Autodesk Inventor part; units mm, degrees
ref_plane "YZ Plane" through (0, 0, 0) normal (1, 0, 0) x (0, 1, 0)
ref_plane "XZ Plane" through (0, 0, 0) normal (0, 1, 0) x (-1, 0, 0)
ref_plane "XY Plane" through (0, 0, 0) normal (0, 0, 1) x (1, 0, 0)
ref_plane "Work Plane1" through (-237.6364, -237.6364, 0) normal (0, 0, 1) x (0.7071, 0.7071, 0)
sketch "Sketch1" plane through (-237.6364, -237.6364, 0) normal (0, 0, 1) x (0.7071, 0.7071, 0)
  circle A0 centre (0, 0) radius 4.15 construction
  circle A1 centre (336.0686, 0) radius 6.45 construction
  circle A2 centre (246.0297, 47.9271) radius 4.83 construction
  circle A3 centre (102, -0.0729) radius 4.83 construction
  circle A4 centre (0, 0) radius 6.8857
  circle A5 centre (336.0686, 0) radius 6.8834
  circle A6 centre (102, -0.0729) radius 6.8834
  circle A7 centre (246.0297, 47.9271) radius 6.8834
  line L0 (78.0149, 71.9271) -> (270.0149, 71.9271) construction
  line L1 (168.0343, 78.2771) -> (168.0343, 71.9271)
  line L2 (168.0343, 78.2771) -> (393.4593, 78.2771)
  line L3 (168.0343, 78.2771) -> (-57.3907, 78.2771)
  line L4 (-57.3907, -31.75) -> (-57.3907, 78.2771)
  line L5 (-57.3907, -31.75) -> (358.1679, -31.75)
  line L6 (393.4593, 3.5414) -> (393.4593, 78.2771)
  arc A8 (358.1679, -31.75) -> (393.4593, 3.5414) centre (358.1679, 3.5414) ccw
  point P0 (336.0686, 0)
  dimension "d0" = 13.7714
  dimension "d1" = 13.7668
  dimension "d2" = 13.7668
  dimension "d3" = 13.7668
  dimension "d6" = 225.425
  dimension "d7" = 225.425
extrude "Extrusion1" add sketch "Sketch1" along normal blind 6.35
sketch "Sketch3" plane through (-237.6364, -237.6364, 6.35) normal (0, 0, 1) x (0.7071, -0.7071, 0)
  circle A0 centre (-63.9271, 166.0149) radius 3.81 construction
  circle A1 centre (-31.9271, 166.0149) radius 3.81 construction
  circle A2 centre (-15.9271, 166.0149) radius 3.81 construction
  circle A3 centre (-63.9271, 86.0149) radius 3.81 construction
  circle A4 centre (16.0729, 166.0149) radius 3.81 construction
  circle A5 centre (-31.9271, 166.0149) radius 3.81 construction
  circle A6 centre (-63.9271, 86.0149) radius 5.08 construction
  circle A7 centre (-31.9271, 86.0149) radius 3.81 construction
  circle A8 centre (-15.9271, 86.0149) radius 3.81 construction
  circle A9 centre (16.0729, 86.0149) radius 3.81 construction
  circle A10 centre (-63.9271, 86.0149) radius 1.778
  circle A11 centre (-31.9271, 166.0149) radius 1.778
  circle A12 centre (-63.9271, 166.0149) radius 1.778
  circle A13 centre (16.0729, 166.0149) radius 1.9304 construction
  circle A14 centre (16.0729, 246.0149) radius 1.9304 construction
  circle A15 centre (-15.9271, 166.0149) radius 1.9304 construction
  circle A16 centre (16.0729, 246.0149) radius 1.778
  point P0 (0, 336.0686)
  dimension "d11" = 3.556
  dimension "d17" = 3.556
  dimension "d18" = 3.556
  dimension "d21" = 3.556
extrude "Extrusion2" cut sketch "Sketch3" against normal through all contours A10 | A11 | A12
properties part number "new sidewall outside"
Part model, mm, in its own coordinate system. Round coordinates to 2 decimals unless told otherwise and drop trailing zeros. Loops run counter-clockwise (first coordinate to the right, second up) from the corner with the lowest first, then second, coordinate; pieces in that order, holes last. Notation, with made-up numbers: (39, 84) -> (75, 84) arc R24 cw to (75, 102) -> close; hole circle Ø7 at (61, 26). An arc over 180 degrees is marked (long way). Use one line per item in the form item = value. Start each with the question number.
Item 1: Band-saw the part on A-A (x = -240). List the corners of the cut face in (y, z), plus the area to 3 significant figures.
Item 2: Two-plate mould, pull along X, no slides. Class faces 1 (the cylindrical face through (-97.855, -36.655, 3.131)), 2 (the flat face through (-176.4, -65.7, 3.1)), 3 (the cylindrical face through (48.41, 18.52, 3.13)): released by +X, released by -X, zero draft, split by the parting line, or undercut.
Item 3: Drop flat-ended pins along their axis: pin 1 Ø2 at (y, z) = (37, 1.5) entering from +X; pin 2 Ø1 at (x, z) = (-126, 1) entering from -Y; pin 3 Ø3 at (x, y) = (-222.02, -131.61) entering from -Z; pin 4 Ø1 at (y, z) = (33.5, 0.5) entering from -X. Give the stop position or say it passes through.
Item 4: Band-saw the part on C-C (y = -205). List the corners of the cut face in (x, z).
Item 5: Drill centre lines: line 1 along Y through (x, z) = (1.5, 3); line 2 along X through (y, z) = (-83.5, 0.5); line 3 along Y through (x, z) = (-288, 5.75). Where is each one in solid material? Low to high.
Item 6: Band-saw the part on B-B (z = 1.5). List the corners of the cut face in (x, y), plus the area to 3 significant figures.
Item 7: Band-saw the part on D-D (x = -191). List the corners of the cut face in (y, z), plus the area to 3 significant figures.
Data:
q1.outline = (-284.9, 0) -> (-244.1, 0) -> (-244.1, 6.35) -> (-284.9, 6.35) -> close; (-231.17, 0) -> (-129.3, 0) -> (-129.3, 6.35) -> (-231.17, 6.35) -> close
q1.area = 906 mm^2
q2.face_1 = undercut
q2.face_2 = released by -X
q2.face_3 = released by +X
q3.pin_1 = 43.56
q3.pin_2 = -171.4
q3.pin_3 = through
q3.pin_4 = -77.7
q4.outline = (-315.7, 0) -> (-160.1, 0) -> (-160.1, 6.35) -> (-315.7, 6.35) -> close
q5.line_1 = -43.4 to -6.72, 6.72 to 79.66
q5.line_2 = -194.2 to -38.6
q5.line_3 = -268.44 to -177.3
q6.outline = (-333.57, -222.87) -> (-255.77, -300.67) -> (38.08, -6.82) arc R35.29 ccw to (38.08, 43.09) -> (-14.77, 95.93) -> close; hole circle Ø13.77 at (-237.64, -237.64); hole circle Ø3.56 at (-222.02, -131.61); hole circle Ø13.77 at (-165.46, -165.56); hole circle Ø3.56 at (-165.45, -75.04); hole circle Ø3.56 at (-142.82, -97.67); hole circle Ø13.77 at (-97.56, -29.78); hole circle Ø13.77 at (0, 0)
q6.area = 48,700 mm^2
q7.outline = (-235.9, 0) -> (-80.3, 0) -> (-80.3, 6.35) -> (-235.9, 6.35) -> close
q7.area = 988 mm^2
